from build123d import *

# Parameters (mm, degrees)
EXTRUDE_THIN1_DEPTH = 90
SKETCH2_R           = 10
BOSS_EXTRUDE1_DEPTH = 90


with BuildPart() as part:
    # Sketch1 → Extrude-Thin1 (new body)
    with BuildSketch(Plane.XY):
        with BuildLine():
            Line((0, -15), (-60, -15))
            ThreePointArc((-60, -15), (-85, -40), (-60, -65))
            Line((-60, -65), (0, -65))
            Line((0, -65), (0, -55))
            Line((0, -55), (-60, -55))
            ThreePointArc((-60, -55), (-75, -40), (-60, -25))
            Line((-60, -25), (0, -25))
            Line((0, -25), (0, -15))
        make_face()
    extrude(amount=EXTRUDE_THIN1_DEPTH)


with BuildPart() as body_2:
    # Sketch2 → Boss-Extrude1 (new body)
    with BuildSketch(Plane(origin=(0, 0, 0), x_dir=(1, 0, 0), z_dir=(0, 1, 0))):
        with BuildLine():
            Line((-85, -25), (-85, -65))
            Line((-85, -65), (-20, -65))
            ThreePointArc((-20, -65), (0, -45), (-20, -25))
            Line((-20, -25), (-85, -25))
        make_face()
        with Locations(Location((-20, -45, 0), (0, 0, 270))):
            Circle(SKETCH2_R, mode=Mode.SUBTRACT)
    extrude(amount=-BOSS_EXTRUDE1_DEPTH)


with BuildPart() as part_1:
    add(part.part)

    # official_combine_multi_inter: union body 2
    add(body_2.part)


solid = part_1.part
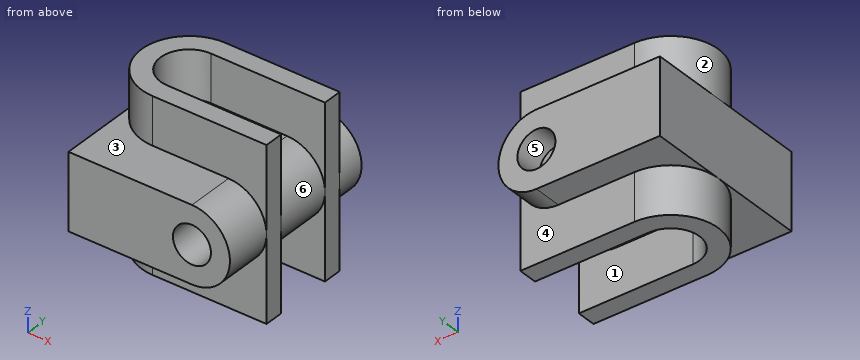
Geometry check sheet. Reference: the model listing, model coordinates, mm. Face numbers are marked on the shaded views. A direction names the side the tool comes from. Give positions to 0.01 mm unless a question says otherwise; leave off trailing zeros. Write each loop counter-clockwise with the first axis right and the second up, starting at its lowest first coordinate (ties: lowest second). Pieces come first, ordered by that corner, then holes. Notation, with made-up numbers: (-30.75, -31.75) - (12.25, -31.75) arc R28 ccw to (12.25, -2.75) - close; hole circle Ø10 at (-14, -4). An arc over 180 degrees is marked (long way). Put each result on its own line as item: value.
1. Draft check along Y on the marked faces 4, 5 and 6. Enter one of: +Y half, -Y half, draft (parallel to the pull), parting line (faces both ways), or undercut.
Ans:
face 4: +Y half
face 5: draft
face 6: undercut
2. Sectioned sample at B-B, the plane z = 23. Enter the section's corners in (x, y).
Ans:
outline: (-60, -65) - (0, -65) - (0, -55) - (-60, -55) arc R15 cw to (-60, -25) - (0, -25) - (0, -15) - (-60, -15) arc R25 ccw to start
3. Sectioned sample at D-D, the plane z = 47.5. Enter the section's corners in (x, y).
Ans:
outline: (-85, -90) - (-29.68, -90) - (-29.68, -65) - (-10.32, -65) - (-10.32, -90) - (-0.16, -90) - (-0.16, -65) - (0, -65) - (0, -55) - (-0.16, -55) - (-0.16, -25) - (0, -25) - (0, -15) - (-0.16, -15) - (-0.16, 0) - (-10.32, 0) - (-10.32, -15) - (-29.68, -15) - (-29.68, 0) - (-85, 0) - close; hole (-29.68, -55) - (-10.32, -55) - (-10.32, -25) - (-29.68, -25) - close
4. Thickness scan on line 1 (X direction, y = -6, z = 45); line 2 (Y direction, x = -30, z = 76); line 3 (Z direction, x = -35.5, y = -29). Record the ranges inside material, lowest first.
Ans:
line 1: x = -85 to -30, -10 to 0
line 2: y = -65 to -55, -25 to -15
line 3: z = 25 to 65
5. Sectioned sample at A-A, the plane y = -69.5. Enter the section's corners in (x, z).
Ans:
outline: (-85, 25) - (-20, 25) arc R20 ccw to (-20, 65) - (-85, 65) - close; hole circle Ø20 at (-20, 45)
6. Set-up check for the marked faces 1, 2 and 3: record each of +Z, -Z, +X, -X, +Y, -Y from which the full face is reachable in a straight line by a thin tool's end or side.
Ans:
face 1: -Z, +X
face 2: +Z, -X
face 3: +Z, -X, -Y
7. Go/stop test with flat-tipped pins: pin 1 (18 mm diameter, centred on x = -20, z = 45, fed in from -Y); pin 2 (13.5 mm diameter, centred on x = -17, z = 76, fed in from +Y); pin 3 (1.5 mm diameter, centred on y = -62, z = 70.5, fed in from -X). Record where each tip stops, or that it passes through.
Ans:
pin 1: stops at y = -65
pin 2: stops at y = -15
pin 3: stops at x = -73.17
8. Sectioned sample at C-C, the plane y = -18. Enter the section's corners in (x, z).
Ans:
outline: (-85, 25) - (-71.87, 25) - (-71.87, 0) - (0, 0) - (0, 90) - (-71.87, 90) - (-71.87, 65) - (-85, 65) - close
